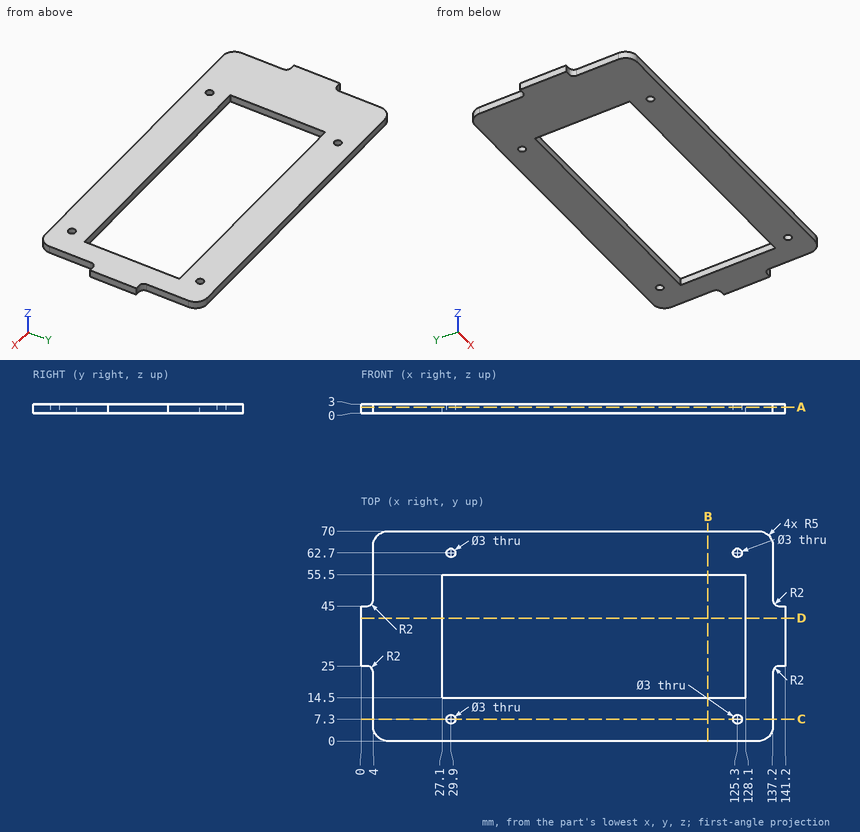
Geometry check sheet. Reference: drawing and pictorial views, mm from the part's lowest x, y, z. Coordinates: 2 decimals unless noted, no trailing zeros. Order: outer loops, then holes, each group sorted by start corner. A loop starts at its lowest first (then second) coordinate and runs counter-clockwise, first axis right, second up. Notation, with made-up numbers: M 57.25,78 L 115.25,78 A24 cw 115.25,114 Z; hole C 78.25,-14 d3. An arc over 180 degrees is marked long. Return JSON: item names as keys, results as strings.
1) Cross-section at B-B, the plane x = 115.5. Record the boundary of the cut face in (y, z).
Answer list:
{"outline": "M 0,0 L 14.5,0 L 14.5,3 L 0,3 Z; M 55.5,0 L 70,0 L 70,3 L 55.5,3 Z"}
2) Gauge pin test, flat ends, axial feed: pin 1 (1.6 mm diameter, centred on x = 140.5, z = 1, fed in from +Y); pin 2 (1 mm diameter, centred on x = 140.5, z = 2, fed in from -Y). Record the tip position at first contact, or that the pin passes through.
Answer list:
{"pin 1": "y = 45", "pin 2": "y = 25"}
3) Cross-section at A-A, the plane z = 1.95. Record the boundary of the cut face in (x, y).
Answer list:
{"outline": "M 0,25 L 2,25 A2 cw 4,23 L 4,5 A5 ccw 9,0 L 132.2,0 A5 ccw 137.2,5 L 137.2,23 A2 cw 139.2,25 L 141.2,25 L 141.2,45 L 139.2,45 A2 cw 137.2,47 L 137.2,65 A5 ccw 132.2,70 L 9,70 A5 ccw 4,65 L 4,47 A2 cw 2,45 L 0,45 Z; hole M 27.1,14.5 L 128.1,14.5 L 128.1,55.5 L 27.1,55.5 Z; hole C 29.9,7.3 d3; hole C 29.9,62.7 d3; hole C 125.3,7.3 d3; hole C 125.3,62.7 d3"}
4) Cross-section at D-D, the plane y = 41. Record the boundary of the cut face in (x, z).
Answer list:
{"outline": "M 0,0 L 27.1,0 L 27.1,3 L 0,3 Z; M 128.1,0 L 141.2,0 L 141.2,3 L 128.1,3 Z"}
5) Cross-section at C-C, the plane y = 7.3. Record the boundary of the cut face in (x, z).
Answer list:
{"outline": "M 4,0 L 28.4,0 L 28.4,3 L 4,3 Z; M 31.4,0 L 123.8,0 L 123.8,3 L 31.4,3 Z; M 126.8,0 L 137.2,0 L 137.2,3 L 126.8,3 Z"}
6) Thickness scan on L1, parallel to Y at x = 125.3, z = 1.35; L2, parallel to X at y = 62.7, z = 0.6; L3, parallel to X at y = 6.5, z = 2.3. Record the ranges inside material, lowest first. Write a range as [from, to].
Answer list:
{"L1": "[0, 5.8], [8.8, 14.5], [55.5, 61.2], [64.2, 70]", "L2": "[4, 28.4], [31.4, 123.8], [126.8, 137.2]", "L3": "[4, 28.63], [31.17, 124.03], [126.57, 137.2]"}
